Can you work these out from the model? Positions are in its coordinate system, mm. A direction names the side the tool comes from. Round coordinates to 2 decimals unless told otherwise and drop trailing zeros. Loops run counter-clockwise (first coordinate to the right, second up) from the corner with the lowest first, then second, coordinate; pieces in that order, holes last. Notation, with made-up numbers: (59.25, 46) -> (86.25, 46) arc R29 ccw to (86.25, 84) -> close; hole circle Ø1 at (-20.5, -35.5). An arc over 180 degrees is marked (long way). Write each question's results on one line, items separated by ' | '.
from build123d import *

# Parameters (mm, degrees)
SKETCH_1_R      = 5
EXTRUDE_1_DEPTH = 7
SKETCH_2_R      = 4
EXTRUDE_2_DEPTH = 1
M4X0_71_D       = 3.3
M4X0_71_DEPTH   = 5.8
M4X0_71_TIP     = 0.991420021
CHAMFER_1_SIZE  = 0.5


with BuildPart() as part:
    # Эскиз1 → Бобышка-Вытянуть1 (new body)
    with BuildSketch(Plane.XY):
        Circle(SKETCH_1_R)
    extrude(amount=EXTRUDE_1_DEPTH)

    # Эскиз2 → Бобышка-Вытянуть2 (add)
    with BuildSketch(Plane.XY.offset(7)):
        Circle(SKETCH_2_R)
    extrude(amount=EXTRUDE_2_DEPTH)

    # Отверстие обработанное метчиком M4x0.71
    with Locations(Plane.XY.offset(8)):
        with Locations((0, 0)):
            Hole(M4X0_71_D / 2, depth=M4X0_71_DEPTH)
            with Locations((0, 0, -(M4X0_71_DEPTH + M4X0_71_TIP / 2))):  # 118° drill point
                Cone(0, M4X0_71_D / 2, M4X0_71_TIP, mode=Mode.SUBTRACT)

    # Фаска1
    chamfer_1_edges = [part.edges().sort_by_distance(p)[0] for p in [
        (-5, 0, 0),
        (-5, 0, 7),
    ]]
    chamfer(chamfer_1_edges, length=CHAMFER_1_SIZE)


solid = part.part
1. On a 3-axis mill with a long thin cutter (end or side, diameter ignored), from which of +Z, -Z, +X, -X, +Y, -Y can I reach the whole of each face in a straight line? I mean faces 1 (the face through (-3, -3, 7)), 2 (the face through (2, 0, 8)). Say none if no direction works.
Final values:
face 1: +Z | face 2: +Z, +X, -X, +Y, -Y
2. We'd pull the mould along Y, two halves only. Please class faces 3 (the face through (1.216, 1.115, 5.059)), 4 (the face through (-0.867, -3.905, 7.493)), 5 (the face through (0, 0, 0)): pulls with the +Y half, pulls with the -Y half, needs draft (parallel to the pull), parting line crosses it, or undercut.
Final values:
face 3: undercut | face 4: parting line crosses it | face 5: needs draft
3. If we section it at A-A (z = 2.5): List the corners of the cut face in (x, y) for me.
Final values:
outline: circle Ø10 at (0, 0); hole circle Ø3.3 at (0, 0)
4. If we section it at B-B (z = 6.75): List the corners of the cut face in (x, y) for me, then the cut area to 3 significant figures.
Final values:
outline: circle Ø9.5 at (0, 0); hole circle Ø3.3 at (0, 0) | area: 62.3 mm2
5. Will these pins go through, and if not, where does the flat tip stop? pin 1 (1.5 mm diameter, centred on y = 1.5, z = 2.5, fed in from -X); pin 2 (4 mm diameter, centred on y = -3.5, z = 4.5, fed in from +X).
Final values:
pin 1: x = -4.94 | pin 2: x = 4.77
6. Please list where these lines run through material, in increasing order: line 1 (Y direction, x = 0, z = 3.9); line 2 (Y direction, x = -1, z = 5.5); line 3 (X direction, y = -0.5, z = 5). Write a range as from..to.
Final values:
line 1: -5..-1.65, 1.65..5 | line 2: -4.9..-1.31, 1.31..4.9 | line 3: -4.97..-1.57, 1.57..4.97
